Print and shaded views of the part. All mm, measured from the part's lowest x, y and z. A direction names the side the tool comes from. Give positions to 0.01 mm unless a question says otherwise; leave off trailing zeros. Loops run counter-clockwise (first coordinate to the right, second up) from the corner with the lowest first, then second, coordinate; pieces in that order, holes last. Notation, with made-up numbers: (-12, 55) -> (6, 55) arc R34 cw to (6, 93) -> close; hole circle Ø9 at (58, 76). An arc over 180 degrees is marked (long way). Answer as a JSON object with one key per item and string values. Group by question number.
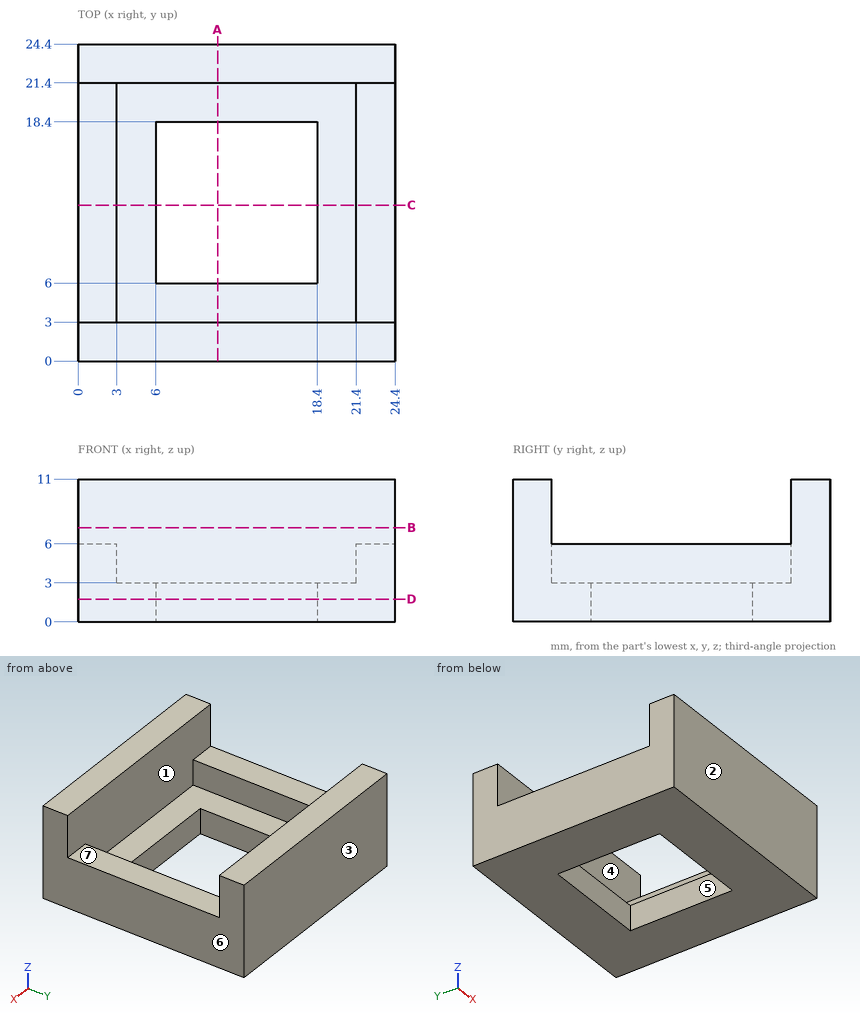
(1) Saw through at C-C on y = 12. List the corners of the cut face in (x, z).
(2) Saw through at D-D on z = 1.75. List the corners of the cut face in (x, y), plus the area to 3 significant figures.
(3) 3-axis set-ups, long thin cutter, end or side, ignore diameter. For the marked faces 4, 5, 6 and 7: which of +Z, -Z, +X, -X, +Y, -Y reach the whole face in a straight line?
(4) Pull direction Y, two halves, no side cores. Call the marked faces 1, 2 and 3: pulls with the +Y half, pulls with the -Y half, needs draft (parallel to the pull), parting line crosses it, or undercut.
(5) Saw through at A-A on x = 10.75. List the corners of the cut face in (y, z), plus the area to 3 significant figures.
(6) Pin check, flat tip, straight feed: pin 1 (2.5 mm diameter, centred on x = 2, y = 9.5, fed in from +Z). Stop position of the tip, or through.
(7) Probe line 1 along Y through (x, z) = (17.75, 0.75); line 2 along Y through (x, z) = (17.5, 5.5). List the from-to ranges inside material, lowest first. Write a range as [from, to].
(8) Saw through at B-B on z = 7.25. List the corners of the cut face in (x, y), plus the area to 3 significant figures.
Calculated:
{
 "1": {"outline": "(0, 0) -> (6, 0) -> (6, 3) -> (3, 3) -> (3, 6) -> (0, 6) -> close; (18.4, 0) -> (24.4, 0) -> (24.4, 6) -> (21.4, 6) -> (21.4, 3) -> (18.4, 3) -> close"},
 "2": {"outline": "(0, 0) -> (24.4, 0) -> (24.4, 24.4) -> (0, 24.4) -> close; hole (6, 6) -> (18.4, 6) -> (18.4, 18.4) -> (6, 18.4) -> close", "area": "442 mm^2"},
 "3": {"face 4": "+Z", "face 5": "+Z, -Z", "face 6": "+Z, -Z, +X, +Y, -Y", "face 7": "+Z, +X, -X"},
 "4": {"face 1": "undercut", "face 2": "pulls with the -Y half", "face 3": "pulls with the +Y half"},
 "5": {"outline": "(0, 0) -> (6, 0) -> (6, 3) -> (3, 3) -> (3, 11) -> (0, 11) -> close; (18.4, 0) -> (24.4, 0) -> (24.4, 11) -> (21.4, 11) -> (21.4, 3) -> (18.4, 3) -> close", "area": "84.0 mm^2"},
 "6": {"pin 1": "stops at z = 6"},
 "7": {"line 1": "y = [0, 6], [18.4, 24.4]", "line 2": "y = [0, 3], [21.4, 24.4]"},
 "8": {"outline": "(0, 0) -> (24.4, 0) -> (24.4, 3) -> (0, 3) -> close; (0, 21.4) -> (24.4, 21.4) -> (24.4, 24.4) -> (0, 24.4) -> close", "area": "146 mm^2"}
}
